Autodesk Inventor part; units mm, degrees
ref_plane "YZ Plane" through (0, 0, 0) normal (1, 0, 0) x (0, 1, 0)
ref_plane "XZ Plane" through (0, 0, 0) normal (0, 1, 0) x (-1, 0, 0)
ref_plane "XY Plane" through (0, 0, 0) normal (0, 0, 1) x (1, 0, 0)
sketch "Эскиз1" plane through (0, 0, 0) normal (0, 1, 0) x (-1, 0, 0)
  line L0 (0, 0) -> (150, 0)
  line L1 (150, 0) -> (150, -150)
  line L2 (150, -150) -> (0, -150)
  line L3 (0, -150) -> (0, 0)
  line L4 (150, 0) -> (137, 0)
  line L5 (137, -8) -> (137, -8)
  line L6 (142, -13) -> (142, -13)
  line L7 (150, -13) -> (150, 0)
  line L8 (150, -150) -> (137, -150)
  line L9 (137, -142) -> (137, -142)
  line L10 (142, -137) -> (142, -137)
  line L11 (150, -137) -> (150, -150)
  line L12 (0, 0) -> (13, 0)
  line L13 (13, -8) -> (13, -8)
  line L14 (8, -13) -> (8, -13)
  line L15 (0, -13) -> (0, 0)
  line L16 (0, -150) -> (13, -150)
  line L17 (13, -142) -> (13, -142)
  line L18 (8, -137) -> (8, -137)
  line L19 (0, -137) -> (0, -150)
  circle A0 centre (143.5, -6.5) radius 2.6
  circle A1 centre (143.5, -143.5) radius 2.6
  circle A2 centre (6.5, -143.5) radius 2.6
  circle A3 centre (6.5, -6.5) radius 2.6
  line L20 (18, -3) -> (132, -3)
  line L21 (147, -18) -> (147, -132)
  line L22 (132, -147) -> (18, -147)
  line L23 (3, -132) -> (3, -18)
  arc A4 (18, -3) -> (13, -8) centre (18, -8) ccw
  arc A5 (8, -13) -> (3, -18) centre (8, -18) ccw
  arc A6 (8, -13) -> (13, -8) centre (8, -8) ccw
  arc A7 (3, -132) -> (8, -137) centre (8, -132) ccw
  arc A8 (13, -142) -> (18, -147) centre (18, -142) ccw
  arc A9 (13, -142) -> (8, -137) centre (8, -142) ccw
  arc A10 (132, -147) -> (137, -142) centre (132, -142) ccw
  arc A11 (142, -137) -> (137, -142) centre (142, -142) ccw
  arc A12 (142, -137) -> (147, -132) centre (142, -132) ccw
  arc A13 (147, -18) -> (142, -13) centre (142, -18) ccw
  arc A14 (137, -8) -> (142, -13) centre (142, -8) ccw
  arc A15 (137, -8) -> (132, -3) centre (132, -8) ccw
  dimension "d0" = 150
  dimension "d1" = 150
  dimension "d11" = 5.2
  dimension "d12" = 5.2
  dimension "d14" = 3
  dimension "d15" = 3
  dimension "d16" = 3
  dimension "d17" = 3
  dimension "d18" = 5
extrude "Выдавливание1" add sketch "Эскиз1" along normal blind 50
extrude "Выдавливание2" add sketch "Эскиз1" against normal blind 3 contours L0 L1 L2 L3 | A0 | A1 | A2 | A3 | L20 A15 A14 A13 L21 A12 A11 A10 L22 A8 A9 A7 L23 A5 A6 A4
sketch "Эскиз2" plane through (0, 50, 0) normal (1, 0, 0) x (0, 0, -1)
  line L0 (147, -50) -> (147, 0)
  line L1 (3, -50) -> (3, 0)
  line L2 (147, 0) -> (3, 0)
  line L3 (3, 0) -> (3, -50)
  line L4 (3, -50) -> (147, -50)
  line L5 (147, -50) -> (147, 0)
  line L6 (147, -50) -> (3, 0)
  line L7 (147, 0) -> (3, -50)
  line L8 (75, -25) -> (75, -35)
  line L9 (25, -33.2281) -> (125, -33.2281)
  line L10 (125, -33.2281) -> (125, -38.2281)
  line L11 (125, -38.2281) -> (25, -38.2281)
  line L12 (25, -38.2281) -> (25, -33.2281)
  line L13 (25, -33.2281) -> (125, -38.2281) construction
  line L14 (125, -33.2281) -> (25, -38.2281) construction
  point P0 (0, -50)
  point P1 (75, -35.7281)
  dimension "d25" = 10
  dimension "d26" = 100
  dimension "d27" = 5
extrude "Выдавливание3" cut sketch "Эскиз2" against normal blind 200 contours L11 L7 L9 L6 | L6 L9 L10 L11 | L11 L12 L9 L7
properties part number "Box"
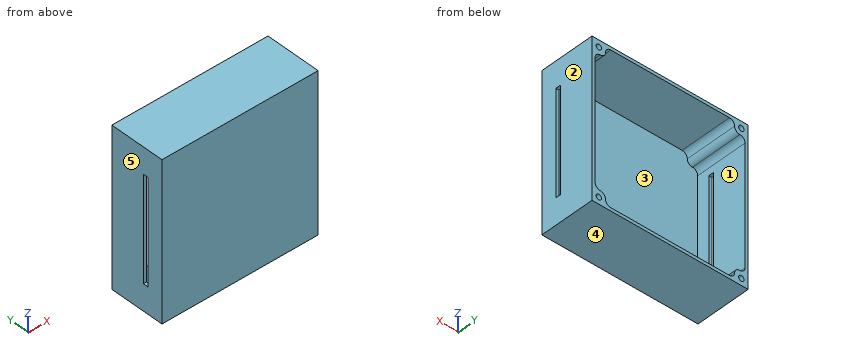
Geometry: final body of the model. Coordinates: model frame, mm. Face numbers are marked on the shaded views. A direction names the side the tool comes from. Coordinates: 2 decimals unless noted, no trailing zeros. Order: outer loops, then holes, each group sorted by start corner. A loop starts at its lowest first (then second) coordinate and runs counter-clockwise, first axis right, second up. Notation, with made-up numbers: (26.25, 80) - (30.25, 80) arc R20 ccw to (30.25, 118) - close; hole circle Ø2 at (-21.75, 74.25). An arc over 180 degrees is marked (long way). Write each question's results on one line, items separated by ' | '.
(1) Line query: line 1 (Z direction, x = -93, y = 30); line 2 (Z direction, x = -7.5, y = 10.5). Output: solid intervals per line, ascending. Write a range as [from, to].
Values found:
line 1: z = [-150, -147], [-3, 0] | line 2: z = [-150, -145.9], [-141.1, -136.97], [-13.03, -8.9], [-4.1, 0]
(2) Mould query, pull axis X, two halves, no side actions, for the marked faces 3, 4 and 5. Classes: +X half, -X half, draft (parallel to the pull), parting line (faces both ways), or undercut.
Values found:
face 3: undercut | face 4: draft | face 5: -X half
(3) Set-up query: the marked faces 1 and 2. Return all of +Z, -Z, +X, -X, +Y, -Y with unobstructed straight access to the full face (end or side cutting, diameter ignored); none if empty.
Values found:
face 1: +Y | face 2: +Z, -Z, +X, +Y, -Y
(4) Section query C-C, the plane y = 23. Return the cut outline in (x, z), plus the area to 3 significant figures.
Values found:
outline: (-150, -150) - (0, -150) - (0, 0) - (-150, 0) - close; hole (-147, -132) arc R5 ccw to (-142, -137) arc R5 cw to (-137, -142) arc R5 ccw to (-132, -147) - (-18, -147) arc R5 ccw to (-13, -142) arc R5 cw to (-8, -137) arc R5 ccw to (-3, -132) - (-3, -18) arc R5 ccw to (-8, -13) arc R5 cw to (-13, -8) arc R5 ccw to (-18, -3) - (-132, -3) arc R5 ccw to (-137, -8) arc R5 cw to (-142, -13) arc R5 ccw to (-147, -18) - close; hole circle Ø5.2 at (-143.5, -143.5); hole circle Ø5.2 at (-143.5, -6.5); hole circle Ø5.2 at (-6.5, -143.5); hole circle Ø5.2 at (-6.5, -6.5) | area: 2,100 mm²
(5) Section query B-B, the plane x = -39. Return the cut outline in (y, z).
Values found:
outline: (-3, -150) - (50, -150) - (50, -147) - (0, -147) - (0, -3) - (50, -3) - (50, 0) - (-3, 0) - close
(6) Section query D-D, the plane z = -11. Return the cut outline in (x, y).
Values found:
outline: (-150, -3) - (0, -3) - (0, 50) - (-12, 50) - (-12, 0) - (-138, 0) - (-138, 50) - (-150, 50) - close
(7) Section query A-A, the plane z = -79. Return the cut outline in (x, y), plus the area to 3 significant figures.
Values found:
outline: (-150, -3) - (0, -3) - (0, 11.77) - (-3, 11.77) - (-3, 0) - (-147, 0) - (-147, 11.77) - (-150, 11.77) - close; (-150, 16.77) - (-147, 16.77) - (-147, 50) - (-150, 50) - close; (-3, 16.77) - (0, 16.77) - (0, 50) - (-3, 50) - close | area: 720 mm²
(8) First-contact query: pin 1 Ø8.5 at (x, z) = (-143.5, -6.5) entering from +Y; pin 2 Ø1.6 at (x, z) = (-144.5, -6) entering from +Y. Flat tips, straight axial feed; report the tip coordinate or a pass-through.
Values found:
pin 1: stops at y = 50 | pin 2: stops at y = 0
